from build123d import *

# Parameters (mm, degrees)
F1_DEPTH  = 304.8
F2_DEPTH  = 304.8
F4_DEPTH  = 304.8
F5_R      = 6.7437
F6_DEPTH  = 6.351
F7_R      = 3.9751
F8_DEPTH  = 292.101
F9_R      = 3.9751
F10_DEPTH = 292.101
F11_R     = 4.7625
F12_DEPTH = 6.351


with BuildPart() as f1:
    # F0 (on Front) → F1 (new body, symmetric)
    with BuildSketch(Plane.XZ):
        Polygon((-12.7, 38.1), (-19.05, 38.1), (-19.05, 0), (19.05, 0), (19.05, 6.35), (-12.7, 6.35), align=None)
    extrude(amount=F1_DEPTH, both=True)

    # F0 (on Front) → F2 (join, symmetric)
    with BuildSketch(Plane.XZ):
        Polygon((-12.7, 38.1), (-19.05, 38.1), (-19.05, 0), (19.05, 0), (19.05, 6.35), (-12.7, 6.35), align=None)
    extrude(amount=F2_DEPTH, both=True)

    # F3 (on Right) → F4 (join, symmetric)
    with BuildSketch(Plane.YZ):
        Polygon((-19.05, 6.35), (-19.05, 0), (19.05, 0), (19.05, 38.1), (12.7, 38.1), (12.7, 6.35), align=None)
    extrude(amount=F4_DEPTH, both=True)

    # F5 (on face) → F6 (cut, through all)
    with BuildSketch(Plane.XY.offset(6.35)):
        with Locations((-279.4, 0)):
            Circle(F5_R)
        with Locations((0, -279.4)):
            Circle(F5_R)
        with Locations((0, 279.4)):
            Circle(F5_R)
        with Locations((279.4, 0)):
            Circle(F5_R)
    extrude(amount=-F6_DEPTH, mode=Mode.SUBTRACT)

    # F7 (on face) → F8 (cut, through all)
    with BuildSketch(Plane.YZ.offset(-12.7)):
        with Locations((295.275, 28.575)):
            Circle(F7_R)
        with Locations((-295.275, 28.575)):
            Circle(F7_R)
    extrude(amount=-F8_DEPTH, mode=Mode.SUBTRACT)

    # F9 (on face) → F10 (cut, through all)
    with BuildSketch(Plane.XZ.offset(-12.7)):
        with Locations((295.275, 28.575)):
            Circle(F9_R)
        with Locations((-295.275, 28.575)):
            Circle(F9_R)
    extrude(amount=-F10_DEPTH, mode=Mode.SUBTRACT)

    # F11 (on face) → F12 (cut, through all)
    with BuildSketch(Plane.XY.offset(6.35)):
        with Locations((0, 184.15)):
            Circle(F11_R)
        with Locations((184.15, 0)):
            Circle(F11_R)
        with Locations((0, -184.15)):
            Circle(F11_R)
        with Locations((-184.15, 0)):
            Circle(F11_R)
    extrude(amount=-F12_DEPTH, mode=Mode.SUBTRACT)


solid = f1.part
Design review of the part built by this model. Coordinates are the model's own, in mm. A direction names the side the tool comes from. Round coordinates to 2 decimals unless told otherwise and drop trailing zeros. Order: outer loops, then holes, each group sorted by start corner. A loop starts at its lowest first (then second) coordinate and runs counter-clockwise, first axis right, second up. Notation, with made-up numbers: M -37,58 L 18,58 A28 ccw 18,95 Z; hole C 55.25,-21 d11. An arc over 180 degrees is marked long. Answer as CSV lines item,"result". Start each with the question number.
1) For pin 1 Ø11.5 at (y, z) = (-184.5, 27) entering from -X; pin 2 Ø12.5 at (x, y) = (184.15, 0) entering from +Z; pin 3 Ø12.5 at (x, z) = (-295.275, 28.575) entering from +Y, all flat-tipped, find the tip position at first contact; note any pin that passes through.
2) Add section B-B (x = 263.5). Give the boundary of the cut face in (y, z).
3) Tool access review of faces 5 (the face through (-13, -304.8, 13)), 6 (the face through (3.625, 285.086, 3.219)), 7 (the face through (148, 12.7, 22)), 8 (the face through (3, 160, 6.35)), 9 (the face through (-160, 12.7, 22)): name each direction out of +Z, -Z, +X, -X, +Y, -Y from which nothing blocks a thin tool from reaching the whole face with its end or side.
4) Wall thickness on line 1 along Y through (x, z) = (0, 3.25); line 2 along Y through (x, z) = (184.15, 2.5); line 3 along X through (y, z) = (11.5, 19): over which ranges is each line inside the solid? List them lowest first. Write a range as [from, to].
5) The part is to be moulded in two halves that separate along X. For faces 1 (the face through (1, -1, 0)), 2 (the face through (-19.05, 160, 19)), 3 (the face through (-12.7, 160, 22)), 4 (the face through (285.83, 2.03, 3.22)), say which applies: +X half, -X half, draft (parallel to the pull), parting line (faces both ways), or undercut.
6) Add section A-A (y = -201). Give the boundary of the cut face in (x, z).
Resolved:
1,pin 1,"x = -19.05"
1,pin 2,"z = 6.35"
1,pin 3,"y = 19.05"
2,outline,"M -19.05,0 L 19.05,0 L 19.05,38.1 L 12.7,38.1 L 12.7,6.35 L -19.05,6.35 Z"
3,face 5,"+Z, -Z, +X, -X, -Y"
3,face 6,"+Z, -Z"
3,face 7,"+Z, +X, -Y"
3,face 8,"+Z, +X, +Y"
3,face 9,"+Z, -X, -Y"
4,line 1,"[-304.8, -286.14], [-272.66, -188.91], [-179.39, 179.39], [188.91, 272.66], [286.14, 304.8]"
4,line 2,"[-19.05, -4.76], [4.76, 19.05]"
4,line 3,"[-19.05, -12.7]"
5,face 1,"draft"
5,face 2,"-X half"
5,face 3,"+X half"
5,face 4,"undercut"
6,outline,"M -19.05,0 L 19.05,0 L 19.05,6.35 L -12.7,6.35 L -12.7,38.1 L -19.05,38.1 Z"
